```python
from build123d import *

# Parameters (mm, degrees)
SKETCH1_R           = 10
BOSS_EXTRUDE7_DEPTH = 14
SKETCH7_W           = 10.45925955
SKETCH7_H           = 19.99905213
BOSS_EXTRUDE9_DEPTH = 80
SKETCH8_W           = 5.913333595
SKETCH8_H           = 12.55111146
CUT_EXTRUDE3_DEPTH  = 55


with BuildPart() as part:
    # Sketch1 → Boss-Extrude7 (new body)
    with BuildSketch(Plane(origin=(0, 0, 0), x_dir=(0, 0, -1), z_dir=(1, 0, 0))):
        Circle(SKETCH1_R)
    extrude(amount=BOSS_EXTRUDE7_DEPTH)

    # Sketch7 → Boss-Extrude9 (add)
    with BuildSketch(Plane(origin=(0, 0, 0), x_dir=(1, 0, 0), z_dir=(0, 1, 0))):
        with Locations((-0.68370382, 0.000473935)):
            Rectangle(SKETCH7_W, SKETCH7_H)
    extrude(amount=BOSS_EXTRUDE9_DEPTH)

    # Sketch8 → Cut-Extrude3 (cut)
    with BuildSketch(Plane(origin=(0, 80, 0), x_dir=(1, 0, 0), z_dir=(0, 1, 0))):
        with Locations((-2.956666798, -0.041837038)):
            Rectangle(SKETCH8_W, SKETCH8_H)
    extrude(amount=-CUT_EXTRUDE3_DEPTH, mode=Mode.SUBTRACT)


solid = part.part
```
Part model, mm, in its own coordinate system. A direction names the side the tool comes from. Give positions to 0.01 mm unless a question says otherwise; leave off trailing zeros. Order: outer loops, then holes, each group sorted by start corner. A loop starts at its lowest first (then second) coordinate and runs counter-clockwise, first axis right, second up. Notation, with made-up numbers: M -3,52 L 4,52 A18 ccw 4,72 Z; hole C 88,88.5 d8. An arc over 180 degrees is marked long. Use a Markdown table: item, result. Add a question column.
(1) Drop flat-ended pins along their axis: P1, Ø1.8, axis at x = -1.5, z = 2.5, coming from the +Y side; P2, Ø4, axis at y = 38.5, z = -4.5, coming from the +X side; P3, Ø11, axis at y = -5, z = -1.5, coming from the -X side; P4, Ø1.8, axis at x = -3, z = 3.5, coming from the -Y side. Give the stop position or say it passes through.
(2) Saw through at C-C, the plane x = 10. Give the cut face in (y, z).
(3) 3-axis set-ups, long thin cutter, end or side, ignore diameter. For faces 4 (the face through (-3, 0, 0)), 5 (the face through (-1, 39, 9.999)), 6 (the face through (-3, 53, 6.317)): which of +Z, -Z, +X, -X, +Y, -Y reach the whole face in a straight line?
(4) Probe line 1 along Z through (x, y) = (-0.25, 33.5); line 2 along X through (y, z) = (35.5, -9); line 3 along X through (y, z) = (69, -1). List the from-to ranges inside material, lowest first. Write a range as [from, to].
(5) Mould opens along Z. For faces 1 (the face through (8.46, -9.76, 2.17)), 2 (the face through (-3, 53, -6.234)), 3 (the face through (0, -4, 0)) say: +Z half, -Z half, draft (parallel to the pull), parting line (faces both ways), or undercut.
(6) Saw through at B-B, the plane y = 69. Give the cut face in (x, z), and give its area (3 significant figures).
(7) Saw through at D-D, the plane z = 7.25. Give the cut face in (x, y).
(8) Saw through at A-A, the plane z = 0. Give the cut face in (x, y).
Answer key:
| question | item | result |
|---|---|---|
| 1 | P1 | y = 25 |
| 1 | P2 | x = 4.55 |
| 1 | P3 | x = -5.91 |
| 1 | P4 | y = 0 |
| 2 | outline | C 0,0 d20 |
| 3 | face 4 | +Z, -Z, -X, -Y |
| 3 | face 5 | +Z, +X, -X, +Y, -Y |
| 3 | face 6 | -X, +Y |
| 4 | line 1 | [-10, -6.23], [6.32, 10] |
| 4 | line 2 | [-5.91, 4.55] |
| 4 | line 3 | [0, 4.55] |
| 5 | face 1 | parting line |
| 5 | face 2 | undercut |
| 5 | face 3 | draft |
| 6 | outline | M -5.91,-10 L 4.55,-10 L 4.55,10 L -5.91,10 L -5.91,6.32 L 0,6.32 L 0,-6.23 L -5.91,-6.23 Z |
| 6 | area | 135 mm^2 |
| 7 | outline | M -5.91,0 L 0,0 L 0,-6.89 L 14,-6.89 L 14,6.89 L 4.55,6.89 L 4.55,80 L -5.91,80 Z |
| 8 | outline | M -5.91,0 L 0,0 L 0,-10 L 14,-10 L 14,10 L 4.55,10 L 4.55,80 L 0,80 L 0,25 L -5.91,25 Z |
